Could you check a few things on this model? Use its own coordinates, in mm. Face numbers are marked on the shaded views. A direction names the side the tool comes from. Give positions to 0.01 mm unless a question says otherwise; leave off trailing zeros. Loops run counter-clockwise (first coordinate to the right, second up) from the corner with the lowest first, then second, coordinate; pieces in that order, holes last. Notation, with made-up numbers: (-18, 67) -> (8, 67) arc R15 cw to (8, 76) -> close; hole circle Ø2 at (-14, 59.5). An arc over 180 degrees is marked (long way). Write each question's results on one line, items separated by ' | '. Start each with the question number.
Q1. Will these pins go through, and if not, where does the flat tip stop? P1, Ø4.5, axis at x = 10, y = -19.5, coming from the +Z side; P2, Ø3, axis at x = -17, y = -9, coming from the -Z side; P3, Ø3, axis at y = 2, z = 1.5, coming from the -X side; P4, Ø1.2, axis at y = -20.5, z = 6, coming from the -X side.
Q2. If I drill on line 1 along X through (y, z) = (0, 3.85); line 2 along Z through (x, y) = (-17.5, -6.5); line 3 along Z through (x, y) = (-3.5, 2.5), over which ranges is the centre line in solid material (lowest first)?
Q3. If we section it at A-A, the plane y = 0: List the corners of the cut face in (x, z) for me.
Q4. If we section it at C-C, the plane z = 4.5: Give the number of separate pieces and of enclosed holes in the cut face, plus the area to 3 significant figures.
Q5. We'd pull the mould along Y, two halves only. Please class the marked faces 3, 4 and 5: released by +Y, released by -Y, zero draft, split by the parting line, or undercut.
Q6. If we section it at B-B, the plane z = 2: List the corners of the cut face in (x, y) for me.
Q7. Which directions (+Z, -Z, +X, -X, +Y, -Y) give clear straight access to the entire face, cutting with the end or side of a thin tool? Please do the marked faces 1 and 2.
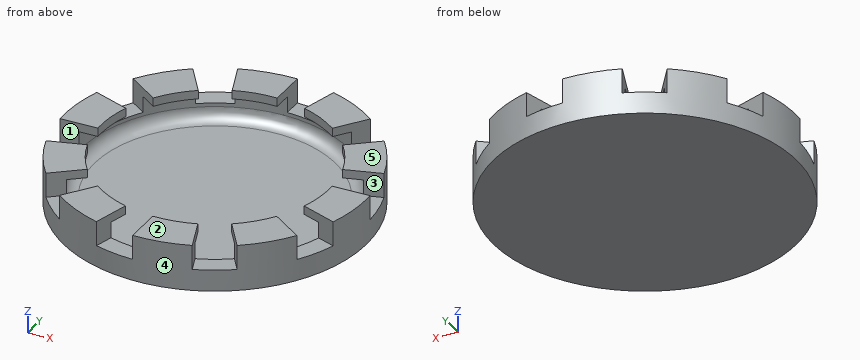
from build123d import *

# Parameters (mm, degrees)
F0_R     = 24.5
F1_DEPTH = 7.5
F2_R     = 21.5
F3_DEPTH = 6.6
F5_R     = 21.5
F5_R_2   = 18.5
F6_DEPTH = 1.4
F8_DEPTH = 4
F9_R     = 2


with BuildPart() as f1:
    # F0 (on Top) → F1 (new body)
    with BuildSketch(Plane.XY):
        Circle(F0_R)
    extrude(amount=F1_DEPTH)

    # F2 (on face) → F3 (cut)
    with BuildSketch(Plane.XY.offset(7.5)):
        Circle(F2_R)
    extrude(amount=-F3_DEPTH, mode=Mode.SUBTRACT)

    # F5 (on offset) → F6 (join, through all)
    with BuildSketch(Plane.XY.offset(6.1)):
        Circle(F5_R)
        Circle(F5_R_2, mode=Mode.SUBTRACT)
    extrude(amount=F6_DEPTH)

    # F7 (on face) → F8 (cut)
    with BuildSketch(Plane.XY.offset(7.5)):
        Polygon((0, 27.140824), (0, 0), (7.272362, 27.140824), align=None)
        Polygon((-15.952976, 21.957388), (0, 0), (-10.069512, 26.231975), align=None)
        Polygon((-25.812457, 8.386976), (0, 0), (-23.565174, 15.303403), align=None)
        Polygon((-25.812457, -8.386976), (0, 0), (-28.059741, -1.470549), align=None)
        Polygon((-15.952976, -21.957388), (0, 0), (-21.83644, -17.682801), align=None)
        Polygon((0, -27.140824), (0, 0), (-7.272362, -27.140824), align=None)
        Polygon((15.952976, -21.957388), (0, 0), (10.069512, -26.231975), align=None)
        Polygon((25.812457, -8.386976), (0, 0), (23.565174, -15.303403), align=None)
        Polygon((25.812457, 8.386976), (0, 0), (28.059741, 1.470549), align=None)
        Polygon((15.952976, 21.957388), (0, 0), (21.83644, 17.682801), align=None)
    extrude(amount=-F8_DEPTH, mode=Mode.SUBTRACT)

    # F9
    f9_edges = [f1.edges().sort_by_distance(p)[0] for p in [
        (-21.5, 0, 0.9),
    ]]
    fillet(f9_edges, radius=F9_R)


solid = f1.part
Final values:
1) P1: stops at z = 3.5 | P2: stops at z = 0 | P3: stops at x = -24.49 | P4: stops at x = -14.29
2) line 1: x = -24.5 to -21.5, 21.5 to 24.5 | line 2: z = 0 to 0.9, 6.1 to 7.5 | line 3: z = 0 to 0.9
3) outline: (-24.5, 0) -> (24.5, 0) -> (24.5, 7.5) -> (18.5, 7.5) -> (18.5, 6.1) -> (21.5, 6.1) -> (21.5, 2.9) arc R2 cw to (19.5, 0.9) -> (-19.5, 0.9) arc R2 cw to (-21.5, 2.9) -> (-21.5, 6.1) -> (-18.5, 6.1) -> (-18.5, 7.5) -> (-24.5, 7.5) -> close
4) separate pieces: 10 | enclosed holes: 0 | area: 253 mm²
5) face 3: undercut | face 4: split by the parting line | face 5: zero draft
6) outline: circle Ø49 at (0, 0); hole circle Ø42.57 at (0, 0)
7) face 1: +Z | face 2: +Z, +X, -X, +Y, -Y
